Design review of the part built by this model. Coordinates are the model's own, in mm. Face numbers are marked on the shaded views. A direction names the side the tool comes from. Round coordinates to 2 decimals unless told otherwise and drop trailing zeros. Loops run counter-clockwise (first coordinate to the right, second up) from the corner with the lowest first, then second, coordinate; pieces in that order, holes last. Notation, with made-up numbers: M 9.25,33.25 L 34.25,33.25 A25 cw 34.25,53.25 Z; hole C 23.25,-7 d7. An arc over 180 degrees is marked long. One line per item, written item: value. Start each with the question number.
Item 1: We need section A-A (x = 0). Write out the cut boundary in (y, z), then the cut area to 3 significant figures.
Item 2: We need section D-D (x = -4.75). Write out the cut boundary in (y, z), then the cut area to 3 significant figures.
Item 3: For line 1 along X through (y, z) = (0, 1); line 2 along Y through (x, z) = (0, 3.05); line 3 along Y through (x, z) = (0, 5.4), list the stretches that pass through material, from the lowest coordinate up.
Item 4: For the marked faces 4 and 5, list the 3-axis set-ups (+Z, -Z, +X, -X, +Y, -Y) from which the entire face can be reached by the end or side of a thin tool; tool diameter is ignored.
Item 5: We need section B-B (y = 0). Write out the cut boundary in (x, z).
Item 6: Mouldability with a two-part tool opening along X and no side actions: class the marked faces 1, 2 and 3 as released by +X, released by -X, zero draft, split by the parting line, or undercut.
Item 7: We need section C-C (z = 1.1). Write out the cut boundary in (x, y), then the cut area to 3 significant figures.
Item 8: Clearance check with flat-ended pins moving along their axes: pin 1 (7.5 mm diameter, centred on x = 0, y = 0, fed in from +Z); pin 2 (1 mm diameter, centred on y = 1.5, z = 1.5, fed in from +X); pin 3 (2 mm diameter, centred on x = 3.5, z = 2.5, fed in from +Y); pin 4 (1.5 mm diameter, centred on x = 1.5, y = -5.5, fed in from -Z). State where each tip first meets the part, or that it passes through.
from build123d import *

# Parameters (mm, degrees)
SKETCH1_R           = 7.7
SKETCH1_R_2         = 3.25
BOSS_EXTRUDE1_DEPTH = 5.85
SKETCH2_R           = 5.25
CUT_EXTRUDE1_DEPTH  = 1.2
SKETCH3_R           = 0.8
CUT_EXTRUDE2_DEPTH  = 10


with BuildPart() as part:
    # Sketch1 → Boss-Extrude1 (new body)
    with BuildSketch(Plane.XY):
        Circle(SKETCH1_R)
        Circle(SKETCH1_R_2, mode=Mode.SUBTRACT)
    extrude(amount=BOSS_EXTRUDE1_DEPTH)

    # Sketch2 → Cut-Extrude1 (cut)
    with BuildSketch(Plane.XY.offset(5.85)):
        Circle(SKETCH2_R)
    extrude(amount=-CUT_EXTRUDE1_DEPTH, mode=Mode.SUBTRACT)

    # Sketch3 → Cut-Extrude2 (cut)
    with BuildSketch(Plane(origin=(0, 0, 0), x_dir=(-1, 0, 0), z_dir=(0, 0, -1))):
        with Locations((0, 7.9)):
            Circle(SKETCH3_R)
    extrude(amount=-CUT_EXTRUDE2_DEPTH, mode=Mode.SUBTRACT)


solid = part.part
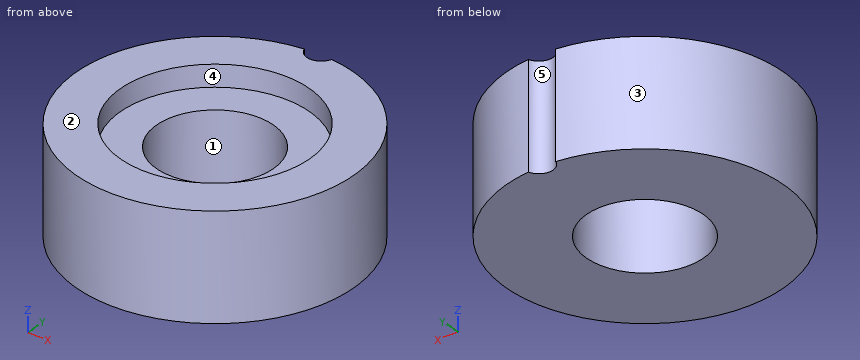
A:
1. outline: M -7.7,0 L -3.25,0 L -3.25,4.65 L -5.25,4.65 L -5.25,5.85 L -7.7,5.85 Z; M 3.25,0 L 7.1,0 L 7.1,5.85 L 5.25,5.85 L 5.25,4.65 L 3.25,4.65 Z
1. area: 43.8 mm2
2. outline: M -6.06,0 L 6.06,0 L 6.06,5.85 L 2.24,5.85 L 2.24,4.65 L -2.24,4.65 L -2.24,5.85 L -6.06,5.85 Z
2. area: 65.5 mm2
3. line 1: -7.7 to -3.25, 3.25 to 7.7
3. line 2: -7.7 to -3.25, 3.25 to 7.1
3. line 3: -7.7 to -5.25, 5.25 to 7.1
4. face 4: +Z
4. face 5: +Z, -Z, +Y
5. outline: M -7.7,0 L -3.25,0 L -3.25,4.65 L -5.25,4.65 L -5.25,5.85 L -7.7,5.85 Z; M 3.25,0 L 7.7,0 L 7.7,5.85 L 5.25,5.85 L 5.25,4.65 L 3.25,4.65 Z
6. face 1: undercut
6. face 2: zero draft
6. face 3: split by the parting line
7. outline: M -0.76,7.66 A7.7 ccw long 0.76,7.66 A0.8 cw Z; hole C 0,0 d6.5
7. area: 152 mm2
8. pin 1: z = 4.65
8. pin 2: x = 7.63
8. pin 3: y = 7.28
8. pin 4: z = 0
